The listing builds one solid part. Answer for the finished solid, in the listing's coordinates (mm). Give positions to 0.01 mm unless a question says otherwise; leave off trailing zeros. Loops run counter-clockwise (first coordinate to the right, second up) from the corner with the lowest first, then second, coordinate; pieces in that order, holes last. Notation, with made-up numbers: (87.25, -18) - (93.25, -18) arc R33 cw to (93.25, 10) - close; hole circle Ø8 at (-4, 57.25). An arc over 180 degrees is marked (long way). Answer as CSV lines item,"result". Start each with the question number.
1) A cutting plane is placed at A-A (x = 18.25). Determine the outline of the cut face in (y, z), and give its area (3 significant figures).
2) Find the intervals of material crossed by line 1 along X through (y, z) = (22.5, 1.8); line 2 along Y through (x, z) = (-23, 0.8); line 3 along Y through (x, z) = (123.25, 1.2), in increasing order.
3) Flat-ended cylindrical pins translate along their axes: pin 1 (1.5 mm diameter, centred on y = 37, z = 1, fed in from +X); pin 2 (1.5 mm diameter, centred on x = 40, y = 15, fed in from -Z). Find the tip coordinate at first contact, or state that the pin passes through.
4) A cutting plane is placed at C-C (y = 40). Determine the outline of the cut face in (x, z), and give its area (3 significant figures).
5) A cutting plane is placed at B-B (z = 1.7). Give the number of separate pieces and of enclosed holes in the cut face, and give its area (3 significant figures).
6) A cutting plane is placed at D-D (x = -32.5). Determine the outline of the cut face in (y, z), and give its area (3 significant figures).
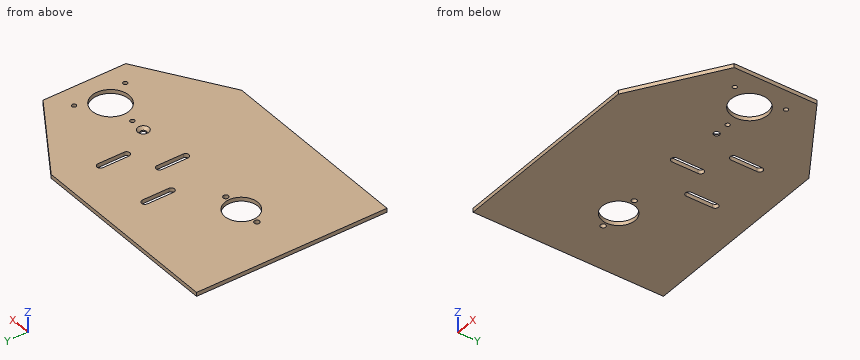
```python
from build123d import *

# Parameters (mm, degrees)
F1_DEPTH        = 3
F3_D            = 28
F5_D            = 3.3
F7_DEPTH        = 3
F9_DEPTH        = 3
F11_D           = 4.5
F11_CSINK_D     = 8.5
F11_CSINK_ANGLE = 90


with BuildPart() as f1:
    # F0 (on Top) → F1 (new body)
    with BuildSketch(Plane.XY):
        Polygon((75, 0), (75, 72.5), (-75, 72.5), (-75, -72.5), (75, -72.5), align=None)
        Polygon((139, 31.5), (75, 72.5), (75, 0), (139, 0), align=None)
        Polygon((139, 0), (75, 0), (75, -72.5), (139, -31.5), align=None)
    extrude(amount=F1_DEPTH)

    # F3 (through all)
    with Locations(Plane.XY.offset(3)):
        with Locations((112, 0)):
            Hole(F3_D / 2)

    # F5 (through all)
    with Locations(Plane.XY.offset(3)):
        with Locations((89.5, 0), (123.25, -19.4855715851), (123.25, 19.4855715851)):
            Hole(F5_D / 2)

    # F6 (on face) → F7 (cut, through all)
    with BuildSketch(Plane.XY.offset(3)):
        with BuildLine():
            Line((-37, 0), (-39, 0))
            Line((-39, 0), (-39, -2))
            ThreePointArc((-39, -2), (-37.5857864376, -1.4142135624), (-37, 0))
        make_face()
        with BuildLine():
            Line((-39, -2), (-39, 0))
            Line((-39, 0), (-37, 0))
            ThreePointArc((-37, 0), (-40.4142135624, 1.4142135624), (-39, -2))
        make_face()
        with BuildLine():
            ThreePointArc((-5, 0), (-7, 2), (-9, 0))
            Line((-9, 0), (-7, 0))
            Line((-7, 0), (-7, -2))
            ThreePointArc((-7, -2), (-5.5857864376, -1.4142135624), (-5, 0))
        make_face()
        with BuildLine():
            Line((-7, 0), (-9, 0))
            ThreePointArc((-9, 0), (-8.4142135624, -1.4142135624), (-7, -2))
            Line((-7, -2), (-7, 0))
        make_face()
        with BuildLine():
            ThreePointArc((-10.5, 0), (-23, 12.5), (-35.5, 0))
            Line((-35.5, 0), (-10.5, 0))
        make_face()
        with BuildLine():
            Line((-10.5, 0), (-35.5, 0))
            ThreePointArc((-35.5, 0), (-23, -12.5), (-10.5, 0))
        make_face()
    extrude(amount=-F7_DEPTH, mode=Mode.SUBTRACT)

    # F8 (on face) → F9 (cut, through all)
    with BuildSketch(Plane.XY.offset(3)):
        with BuildLine():
            Line((38.75, 15), (38.75, -5))
            ThreePointArc((38.75, -5), (41.25, -7.5), (43.75, -5))
            Line((43.75, -5), (43.75, 15))
            ThreePointArc((43.75, 15), (41.25, 17.5), (38.75, 15))
        make_face()
        with BuildLine():
            ThreePointArc((61.75, 23), (62.482233047, 21.232233047), (64.25, 20.5))
            Line((64.25, 20.5), (64.25, 45.5))
            ThreePointArc((64.25, 45.5), (62.482233047, 44.767766953), (61.75, 43))
            Line((61.75, 43), (61.75, 23))
        make_face()
        with BuildLine():
            Line((64.25, 45.5), (64.25, 20.5))
            ThreePointArc((64.25, 20.5), (66.017766953, 21.232233047), (66.75, 23))
            Line((66.75, 23), (66.75, 43))
            ThreePointArc((66.75, 43), (66.017766953, 44.767766953), (64.25, 45.5))
        make_face()
        with BuildLine():
            Line((20.75, 23), (20.75, 43))
            ThreePointArc((20.75, 43), (18.25, 45.5), (15.75, 43))
            Line((15.75, 43), (15.75, 23))
            ThreePointArc((15.75, 23), (18.25, 20.5), (20.75, 23))
        make_face()
    extrude(amount=-F9_DEPTH, mode=Mode.SUBTRACT)

    # F11 (through all)
    with Locations(Plane.XY.offset(3)):
        with Locations((78.15, 0)):
            CounterSinkHole(F11_D / 2, F11_CSINK_D / 2, counter_sink_angle=F11_CSINK_ANGLE)


solid = f1.part
```
Ans:
1,outline,"(-72.5, 0) - (20.5, 0) - (20.5, 3) - (-72.5, 3) - close; (45.5, 0) - (72.5, 0) - (72.5, 3) - (45.5, 3) - close"
1,area,"360 mm2"
2,line 1,"-75 to 15.8, 20.7 to 61.8, 66.7 to 139"
2,line 2,"-72.5 to -12.5, 12.5 to 72.5"
2,line 3,"-41.59 to -21.14, -17.84 to -8.33, 8.33 to 17.84, 21.14 to 41.59"
3,pin 1,"x = 131.59"
3,pin 2,"through"
4,outline,"(-75, 0) - (15.75, 0) - (15.75, 3) - (-75, 3) - close; (20.75, 0) - (61.75, 0) - (61.75, 3) - (20.75, 3) - close; (66.75, 0) - (125.73, 0) - (125.73, 3) - (66.75, 3) - close"
4,area,"572 mm2"
5,separate pieces,"1"
5,enclosed holes,"11"
5,area,"26,900 mm2"
6,outline,"(-72.5, 0) - (-8.12, 0) - (-8.12, 3) - (-72.5, 3) - close; (8.12, 0) - (72.5, 0) - (72.5, 3) - (8.12, 3) - close"
6,area,"386 mm2"
